from build123d import *

# Parameters (mm, degrees)
F1_DEPTH  = 10
F2_W      = 30
F2_H      = 25
F3_DEPTH  = 5
F4_W      = 30
F4_H      = 20
F5_DEPTH  = 5
F6_W      = 25
F6_H      = 13
F7_DEPTH  = 13
F8_R      = 2.1
F9_DEPTH  = 6
F11_DEPTH = 25
F12_R     = 1.75
F12_R_2   = 2.1
F13_DEPTH = 25


with BuildPart() as f1:
    # F0 (on Top) → F1 (new body)
    with BuildSketch(Plane.XY):
        Polygon((15, 12.5), (-15, 12.5), (-15, -12.5), (-40, -12.5), (-68.291549, -105.862112), (-75.867307, -105.862112), (-75.867307, -130.862112), (-90, -177.5), (90, -177.5), (75.867307, -130.862112), (75.867307, -105.862112), (68.291549, -105.862112), (40, -12.5), (15, -12.5), align=None)
        Polygon((-10, -157.5), (-68.265812, -157.5), (-38.036853, -57.744435), align=None, mode=Mode.SUBTRACT)
        Polygon((68.265812, -157.5), (10, -157.5), (38.319605, -58.677516), align=None, mode=Mode.SUBTRACT)
        Polygon((0, -113.740444), (-22.281395, -34.462891), (22.718605, -34.462891), align=None, mode=Mode.SUBTRACT)
    extrude(amount=F1_DEPTH)

    # F2 (on face) → F3 (cut)
    with BuildSketch(Plane(origin=(0, 0, 0), x_dir=(1, 0, 0), z_dir=(0, 0, -1))):
        Rectangle(F2_W, F2_H)
    extrude(amount=-F3_DEPTH, mode=Mode.SUBTRACT)

    # F4 (on face) → F5 (cut)
    with BuildSketch(Plane.XY.offset(10)):
        with Locations((-30, -22.5)):
            Rectangle(F4_W, F4_H)
        with Locations((30, -22.5)):
            Rectangle(F4_W, F4_H)
    extrude(amount=-F5_DEPTH, mode=Mode.SUBTRACT)

    # F6 (on face) → F7 (join)
    with BuildSketch(Plane.XY.offset(10)):
        with Locations((-67.5, -171)):
            Rectangle(F6_W, F6_H)
        with Locations((0, -171)):
            Rectangle(F6_W, F6_H)
        with Locations((67.5, -171)):
            Rectangle(F6_W, F6_H)
    extrude(amount=-F7_DEPTH)

    # F8 (on face) → F9 (cut)
    with BuildSketch(Plane(origin=(0, 0, -3), x_dir=(1, 0, 0), z_dir=(0, 0, -1))):
        with Locations((-74, 171)):
            Circle(F8_R)
        with Locations((-61, 171)):
            Circle(F8_R)
        with Locations((-6.5, 171)):
            Circle(F8_R)
        with Locations((6.5, 171)):
            Circle(F8_R)
        with Locations((61, 171)):
            Circle(F8_R)
        with Locations((74, 171)):
            Circle(F8_R)
    extrude(amount=-F9_DEPTH, mode=Mode.SUBTRACT)

    # F10 (on face) → F11 (cut)
    with BuildSketch(Plane(origin=(0, 0, 5), x_dir=(1, 0, 0), z_dir=(0, 0, -1))):
        Polygon((-15, 32.5), (-15, -12.5), (-12, -12.5), align=None)
        Polygon((12, -12.5), (15, -12.5), (15, 32.5), align=None)
    extrude(amount=-F11_DEPTH, mode=Mode.SUBTRACT)

    # F12 (on face) → F13 (cut)
    with BuildSketch(Plane(origin=(0, 0, 0), x_dir=(1, 0, 0), z_dir=(0, 0, -1))):
        with Locations((0, -5.5)):
            Circle(F12_R)
        with Locations((-8, 5.5)):
            Circle(F12_R)
        with Locations((8, 5.5)):
            Circle(F12_R)
        with Locations((32, 26.462891)):
            Circle(F12_R_2)
        with Locations((23, 18.5)):
            Circle(F12_R_2)
        with Locations((-23, 26.462891)):
            Circle(F12_R_2)
        with Locations((-32, 18.5)):
            Circle(F12_R_2)
    extrude(amount=-F13_DEPTH, mode=Mode.SUBTRACT)


solid = f1.part
Here's how the part is built. I have some questions about the finished solid (model axes, mm). A direction names the side the tool comes from. Give positions to 0.01 mm unless a question says otherwise; leave off trailing zeros. Loops run counter-clockwise (first coordinate to the right, second up) from the corner with the lowest first, then second, coordinate; pieces in that order, holes last. Notation, with made-up numbers: (-23.75, 36) -> (9.25, 36) arc R28 ccw to (9.25, 54) -> close; hole circle Ø4 at (-35, 3.25). An arc over 180 degrees is marked (long way). Answer as a JSON object with one key per item and string values. Group by question number.
Item 1: On a 3-axis mill with a long thin cutter (end or side, diameter ignored), from which of +Z, -Z, +X, -X, +Y, -Y can I reach the whole of each face in a straight line? I mean faces 1 (the flat face through (0, -34.463, 5)), 2 (the cylindrical face through (-74.273, -173.082, -0.042)), 3 (the flat face through (30, -32.5, 8)). Say none if no direction works.
Item 2: Imagine slicing it at B-B on y = -151. Write out the boundary of the cut face in (x, z), then the cut area to 3 significant figures.
Item 3: I need wall thicknesses on L1, parallel to Z at x = -16.5, y = -162; L2, parallel to X at y = -5.5, z = 7.85; L3, parallel to X at y = -120.5, z = 9.5. Which ranges of each line are inside material? Lowest first, please.
Item 4: Thinking about a two-plate mould opening in Y: for faces 4 (the flat face through (67, -171, -3)), 5 (the flat face through (54.344, -59.835, 4.93)), 6 (the cylindrical face through (-21.871, -28.234, 2.465)), which applies, pulls with the +Y half, pulls with the -Y half, needs draft (parallel to the pull), parting line crosses it, or undercut?
Item 5: Imagine slicing it at A-A on x = -51.5. Write out the boundary of the cut face in (y, z).
Item 6: Imagine slicing it at C-C on y = -89.5. Write out the boundary of the cut face in (x, z), then the cut area to 3 significant figures.
Item 7: Will these pins go through, and if not, where does the flat tip stop? pin 1 (4 mm diameter, centred on x = -27, y = -32.5, fed in from -Z); pin 2 (4 mm diameter, centred on y = -35.5, z = 0, fed in from -X); pin 3 (1.7 mm diameter, centred on y = -30.5, z = 7.5, fed in from +X).
Answer list:
{
 "1": {"face 1": "+Z, -Z", "face 2": "-Z", "face 3": "+Z, +Y"},
 "2": {"outline": "(-81.97, 0) -> (-66.3, 0) -> (-66.3, 10) -> (-81.97, 10) -> close; (-11.83, 0) -> (11.86, 0) -> (11.86, 10) -> (-11.83, 10) -> close; (66.3, 0) -> (81.97, 0) -> (81.97, 10) -> (66.3, 10) -> close", "area": "550 mm2"},
 "3": {"L1": "z = 0 to 10", "L2": "x = -13.2 to -9.75, -6.25 to 6.25, 9.75 to 13.2", "L3": "x = -75.87 to -57.05, -20.4 to 20.6, 57.05 to 75.87"},
 "4": {"face 4": "needs draft", "face 5": "pulls with the +Y half", "face 6": "undercut"},
 "5": {"outline": "(-177.5, 0) -> (-157.5, 0) -> (-157.5, 10) -> (-177.5, 10) -> close; (-102.17, 0) -> (-50.45, 0) -> (-50.45, 10) -> (-102.17, 10) -> close"},
 "6": {"outline": "(-63.33, 0) -> (-47.66, 0) -> (-47.66, 10) -> (-63.33, 10) -> close; (-29.11, 0) -> (-6.81, 0) -> (-6.81, 10) -> (-29.11, 10) -> close; (6.95, 0) -> (29.49, 0) -> (29.49, 10) -> (6.95, 10) -> close; (47.66, 0) -> (63.33, 0) -> (63.33, 10) -> (47.66, 10) -> close", "area": "762 mm2"},
 "7": {"pin 1": "stops at z = 0", "pin 2": "stops at x = -47.58", "pin 3": "stops at x = 45.71"}
}
